Can you work these out from the model? Positions are in its coordinate system, mm. Face numbers are marked on the shaded views. A direction names the side the tool comes from. Coordinates: 2 decimals unless noted, no trailing zeros. Order: outer loops, then holes, each group sorted by start corner. A loop starts at its lowest first (then second) coordinate and runs counter-clockwise, first axis right, second up. Notation, with made-up numbers: (-18.75, 83.25) - (2.25, 83.25) arc R4 ccw to (2.25, 88.25) - close; hole circle Ø6 at (6, 30). An arc over 180 degrees is marked (long way). Use a Markdown table: item, result. Add a question column.
(1) We'd pull the mould along Z, two halves only. Please class the marked faces 1, 2 and 3: pulls with the +Z half, pulls with the -Z half, needs draft (parallel to the pull), parting line crosses it, or undercut.
(2) On a 3-axis mill with a long thin cutter (end or side, diameter ignored), from which of +Z, -Z, +X, -X, +Y, -Y can I reach the whole of each face in a straight line? I mean the marked faces 4, 5 and 6. Say none if no direction works.
(3) If I drill on L1, parallel to Z at x = 34.5, y = -27.5; L2, parallel to X at y = -26, z = 2.5; L3, parallel to Y at x = -27, z = -34, over which ranges is the centre line in solid material (lowest first)? Write a range as [from, to].
(4) I want a section at C-C (y = -24). List the corners of the cut face in (x, z) for me.
(5) I want a section at B-B (x = 60). List the corners of the cut face in (y, z) for me, and give its area (3 significant figures).
(6) I want a section at D-D (z = 0). List the corners of the cut face in (x, y) for me.
(7) For pin 1 Ø14 at (x, y) = (-37, -7) entering from -Z; pin 2 Ø1.7 at (y, z) = (-9, -33.5) entering from +X; pin 3 Ø8 at (x, y) = (56, -44) entering from -Z, each with a flat end and sliding along its axis, tell me the tip position at first contact or that it passes through.
(8) I want a section at A-A (y = -6.5). List the corners of the cut face in (x, z) for me, and give its area (3 significant figures).
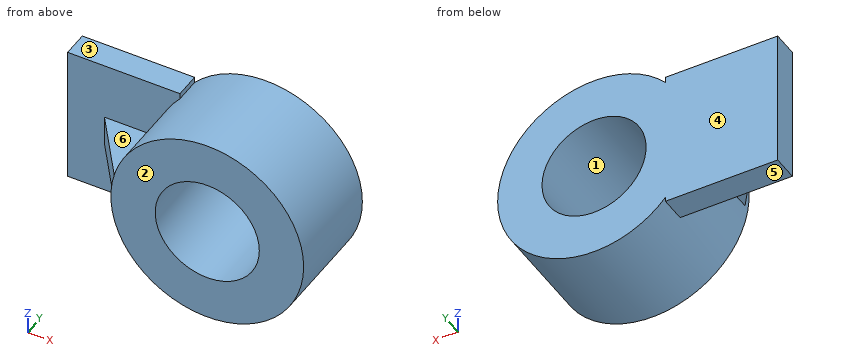
```python
from build123d import *

# Parameters (mm, degrees)
F1_R          = 48.010514
F2_DEPTH      = 50.8
F0_W          = 55.918477
F0_H          = 69.615215
F5_DEPTH      = 12.7
F6_R          = 25.926633
F3_DEPTH      = 50.801
F4_DEPTH      = 6.352296
F4_DEPTH_BACK = 8.470742


with BuildPart() as f2:
    # F1 (on Front) → F2 (new body)
    with BuildSketch(Plane.XZ):
        with Locations((35.529003, 0)):
            Circle(F1_R)
    extrude(amount=F2_DEPTH)

    # F0 (on Front) → F5 (join)
    with BuildSketch(Plane.XZ):
        with Locations((-27.959238, 0.355854)):
            Rectangle(F0_W, F0_H)
    extrude(amount=F5_DEPTH)

    # F6 (on face) → F3 (cut, through all)
    with BuildSketch(Plane.XZ.offset(50.8)):
        with Locations((35.529003, 0)):
            Circle(F6_R)
    extrude(amount=-F3_DEPTH, mode=Mode.SUBTRACT)

    # F7 (on Top) → F4 (join, two sides)
    with BuildSketch(Plane.XY) as f4_sk:
        Polygon((-37.657067, -12.615045), (-12.744168, -46.766188), (-12.455202, -12.37454), align=None)
    extrude(amount=F4_DEPTH)
    extrude(f4_sk.sketch, amount=-F4_DEPTH_BACK)


solid = f2.part
```
Answers follow:
| question | item | result |
|---|---|---|
| 1 | face 1 | undercut |
| 1 | face 2 | needs draft |
| 1 | face 3 | pulls with the +Z half |
| 2 | face 4 | +Z, -Z, +X, -X, +Y |
| 2 | face 5 | -Z, -X, +Y, -Y |
| 2 | face 6 | +Z, -X, -Y |
| 3 | L1 | z = [-48, -25.91], [25.91, 48] |
| 3 | L2 | x = [-27.89, -12.57], [-12.42, 9.72], [61.33, 83.47] |
| 3 | L3 | y = [-12.7, 0] |
| 4 | outline | (-29.35, -8.47) - (-12.55, -8.47) - (-12.55, 6.35) - (-29.35, 6.35) - close; circle Ø96.02 at (35.53, 0); hole circle Ø51.85 at (35.53, 0) |
| 5 | outline | (-50.8, -41.31) - (0, -41.31) - (0, -8.57) - (-50.8, -8.57) - close; (-50.8, 8.57) - (0, 8.57) - (0, 41.31) - (-50.8, 41.31) - close |
| 5 | area | 3,330 mm² |
| 6 | outline | (-55.92, -12.7) - (-37.6, -12.7) - (-12.74, -46.77) - (-12.48, -15.51) - (-12.48, -50.8) - (9.6, -50.8) - (9.6, 0) - (-55.92, 0) - close; (61.46, -50.8) - (83.54, -50.8) - (83.54, 0) - (61.46, 0) - close |
| 7 | pin 1 | stops at z = -34.45 |
| 7 | pin 2 | stops at x = 70.73 |
| 7 | pin 3 | stops at z = -45.1 |
| 8 | outline | (-55.92, -34.45) - (0, -34.45) - (0, -32.29) arc R48.01 ccw (long way) to (0, 32.29) - (0, 35.16) - (-55.92, 35.16) - close; hole circle Ø51.85 at (35.53, 0) |
| 8 | area | 8,470 mm² |
